Could you check a few things on this drawing? It's one solid part, dimensions in mm from its lowest x, y, z. Give positions to 0.01 mm unless a question says otherwise; leave off trailing zeros. Loops run counter-clockwise (first coordinate to the right, second up) from the corner with the lowest first, then second, coordinate; pieces in that order, holes last. Notation, with made-up numbers: (22, 37.5) - (58, 37.5) arc R8 ccw to (58, 42.5) - close; hole circle Ø5 at (65, 12). An arc over 180 degrees is marked (long way). Use a Markdown table: item, result.
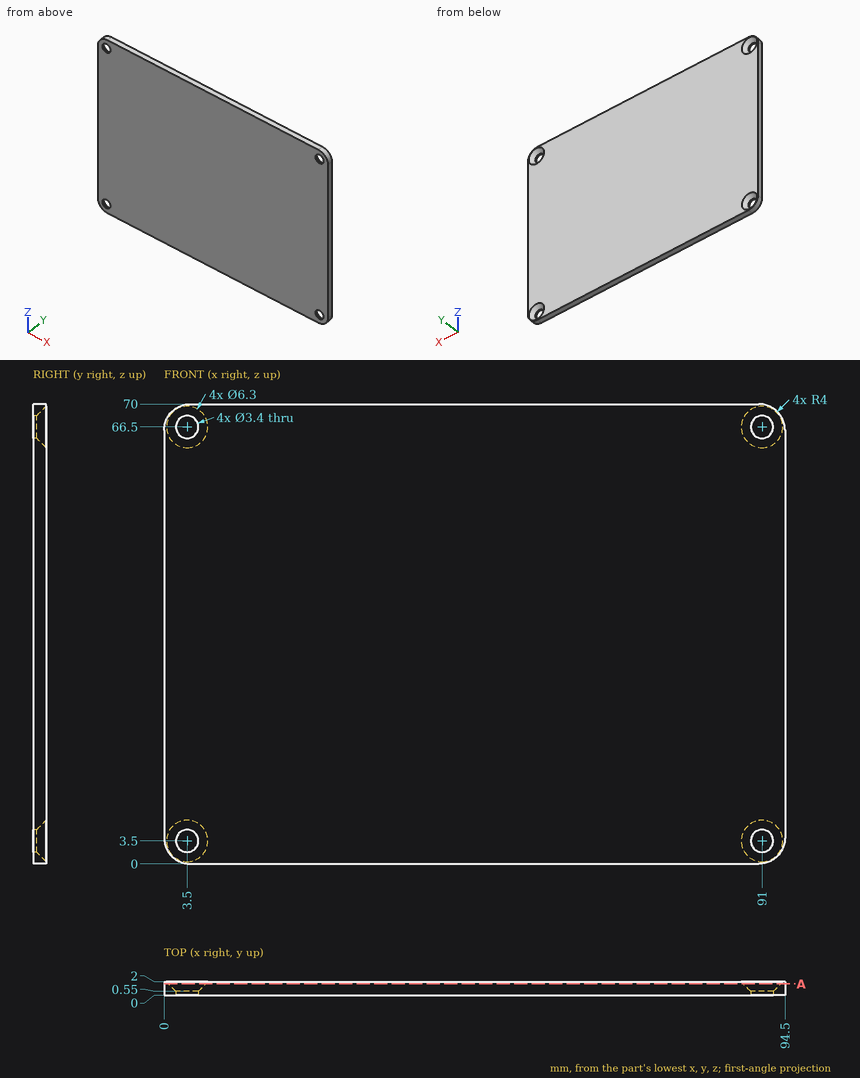
(1) Suppose I cut it at A-A on y = 1.7. Write out the boundary of the cut face in (x, z), plus the area to 3 significant figures.
A:
| item | result |
|---|---|
| outline | (0, 4) arc R4 ccw to (4, 0) - (90.5, 0) arc R4 ccw to (94.5, 4) - (94.5, 66) arc R4 ccw to (90.5, 70) - (4, 70) arc R4 ccw to (0, 66) - close; hole circle Ø5.7 at (3.5, 3.5); hole circle Ø5.7 at (3.5, 66.5); hole circle Ø5.7 at (91, 3.5); hole circle Ø5.7 at (91, 66.5) |
| area | 6,500 mm2 |
(2) If I drill on line 1 (X direction, y = 0.2, z = 66.5); line 2 (Z direction, x = 3.5, y = 0.45), over which ranges is the centre line in solid material (lowest first)?
A:
| item | result |
|---|---|
| line 1 | 0.03 to 1.8, 5.2 to 89.3, 92.7 to 94.47 |
| line 2 | 0.03 to 1.8, 5.2 to 64.8, 68.2 to 69.97 |
(3) Will this pin go through, and if not, where does the flat tip stop? pin 1 (4.5 mm diameter, centred on x = 3.5, z = 66.5, fed in from +Y).
A:
| item | result |
|---|---|
| pin 1 | y = 1.1 |
